For this review, take the finished solid that the model builds, in its own axes (mm). A direction names the side the tool comes from. Coordinates: 2 decimals unless noted, no trailing zeros. Order: outer loops, then holes, each group sorted by start corner. A loop starts at its lowest first (then second) coordinate and runs counter-clockwise, first axis right, second up. Notation, with made-up numbers: (58.25, -24) -> (107.25, -24) arc R19 cw to (107.25, -19) -> close; hole circle Ø4 at (25, 36.5). An arc over 180 degrees is marked (long way). Answer as a JSON object with one key per item and string values. Group by question number.
1) Wall thickness on L1, parallel to X at y = 16, z = 112; L2, parallel to Y at x = 186.75, z = 135.5; L3, parallel to Z at x = 184.25, y = 3: over which ranges is each line inside the solid? List them lowest first.
2) Add section A-A, the plane x = 185. Write out the cut boundary in (y, z).
3) Machinability: for faces 4 (the flat face through (182, 22, 130)), 5 (the flat face through (184, -17, 119)), 6 (the flat face through (185.6, -19.5, 129.3)), which of the approach directions +Z, -Z, +X, -X, +Y, -Y give a long, thin tool a straight path to every point of the face, cutting with its end or side? Answer none if there is none.
4) Draft analysis for pull direction Y (two halves, no side actions). For faces 1 (the flat face through (184, 17, 119)), 2 (the flat face through (182, -22, 130)), 3 (the flat face through (184, -21, 115.5)), state which applies: +Y half, -Y half, draft (parallel to the pull), parting line (faces both ways), or undercut.
5) Add section B-B, the plane z = 114. Write out the cut boundary in (x, y).
6) For pin 1 (1.2 mm diameter, centred on y = -16.5, z = 140, fed in from +X); pin 2 (0.8 mm diameter, centred on x = 186.5, z = 136.5, fed in from +Y); pin 3 (12 mm diameter, centred on y = 10, z = 142, fed in from +X); pin 4 (5.5 mm diameter, centred on x = 197, y = 16, fed in from -Z), all flat-tipped, find the tip position at first contact; note any pin that passes through.
7) Add section D-D, the plane z = 119.5. Write out the cut boundary in (x, y), then the cut area to 3 significant figures.
8) Add section C-C, the plane y = -16.5. Write out the cut boundary in (x, z).
from build123d import *

# Parameters (mm, degrees)
MOUNTING_FOOT_SKETCH_W      = 24
MOUNTING_FOOT_SKETCH_H      = 46
MOUNTING_FOOT_DEPTH         = 3
BACK_PLATE_SKETCH_W         = 3
BACK_PLATE_SKETCH_H         = 44
BACK_PLATE_DEPTH            = 31.5
CLIP_RAILS_DEPTH            = 30
TOP_RETAINING_RAIL_SKETCH_W = 6.1
TOP_RETAINING_RAIL_SKETCH_H = 40
TOP_RETAINING_RAIL_DEPTH    = 2
PCB_SUPPORT_SKETCH_R        = 2
PCB_SUPPORTS_DEPTH          = 3
MOUNTING_HOLES_SKETCH_R     = 1.7
MOUNTING_HOLES_DEPTH        = 3.2


with BuildPart() as part:
    # Mounting Foot Sketch → Mounting Foot (new body)
    with BuildSketch(Plane.XY.offset(111.5)):
        with Locations((190, 0)):
            Rectangle(MOUNTING_FOOT_SKETCH_W, MOUNTING_FOOT_SKETCH_H)
    extrude(amount=MOUNTING_FOOT_DEPTH)

    # Back Plate Sketch → Back Plate (add)
    with BuildSketch(Plane.XY.offset(114.5)):
        with Locations((179.5, 0)):
            Rectangle(BACK_PLATE_SKETCH_W, BACK_PLATE_SKETCH_H)
    extrude(amount=BACK_PLATE_DEPTH)

    # Clip Rail Sketch → Clip Rails (add)
    with BuildSketch(Plane.XY.offset(115.5)):
        Polygon((181, -22), (187.1, -22), (187.1, -19), (185.6, -19), (185.6, -20), (181, -20), align=None)
        Polygon((181, 20), (185.6, 20), (185.6, 19), (187.1, 19), (187.1, 22), (181, 22), align=None)
    extrude(amount=CLIP_RAILS_DEPTH)

    # Top Retaining Rail Sketch → Top Retaining Rail (add)
    with BuildSketch(Plane.XY.offset(143.5)):
        with Locations((184.05, 0)):
            Rectangle(TOP_RETAINING_RAIL_SKETCH_W, TOP_RETAINING_RAIL_SKETCH_H)
    extrude(amount=TOP_RETAINING_RAIL_DEPTH)

    # PCB Support Sketch → PCB Supports (add)
    with BuildSketch(Plane(origin=(181, 0, 0), x_dir=(0, 0, -1), z_dir=(1, 0, 0))):
        with Locations(Location((-119.5, -17, 0), (0, 0, 180))):
            Circle(PCB_SUPPORT_SKETCH_R)
        with Locations(Location((-140.5, -17, 0), (0, 0, 180))):
            Circle(PCB_SUPPORT_SKETCH_R)
        with Locations(Location((-119.5, 17, 0), (0, 0, 180))):
            Circle(PCB_SUPPORT_SKETCH_R)
        with Locations(Location((-140.5, 17, 0), (0, 0, 180))):
            Circle(PCB_SUPPORT_SKETCH_R)
    extrude(amount=PCB_SUPPORTS_DEPTH)

    # Mounting Holes Sketch → Mounting Holes (cut)
    with BuildSketch(Plane.XY.offset(111.4)):
        with Locations((185, -16)):
            Circle(MOUNTING_HOLES_SKETCH_R)
        with Locations((185, 16)):
            Circle(MOUNTING_HOLES_SKETCH_R)
        with Locations((197, -16)):
            Circle(MOUNTING_HOLES_SKETCH_R)
        with Locations((197, 16)):
            Circle(MOUNTING_HOLES_SKETCH_R)
    extrude(amount=MOUNTING_HOLES_DEPTH, mode=Mode.SUBTRACT)


solid = part.part
Output values:
{
 "1": {"L1": "x = 178 to 183.3, 186.7 to 195.3, 198.7 to 202", "L2": "y = -22 to -19, 19 to 22", "L3": "z = 111.5 to 114.5, 143.5 to 145.5"},
 "2": {"outline": "(-23, 111.5) -> (-17.7, 111.5) -> (-17.7, 114.5) -> (-23, 114.5) -> close; (-22, 115.5) -> (-20, 115.5) -> (-20, 143.5) -> (20, 143.5) -> (20, 115.5) -> (22, 115.5) -> (22, 145.5) -> (-22, 145.5) -> close; (-14.3, 111.5) -> (14.3, 111.5) -> (14.3, 114.5) -> (-14.3, 114.5) -> close; (17.7, 111.5) -> (23, 111.5) -> (23, 114.5) -> (17.7, 114.5) -> close"},
 "3": {"face 4": "+Z, +X, -X, +Y", "face 5": "+X", "face 6": "none"},
 "4": {"face 1": "undercut", "face 2": "-Y half", "face 3": "draft"},
 "5": {"outline": "(178, -23) -> (202, -23) -> (202, 23) -> (178, 23) -> close; hole circle Ø3.4 at (185, -16); hole circle Ø3.4 at (185, 16); hole circle Ø3.4 at (197, -16); hole circle Ø3.4 at (197, 16)"},
 "6": {"pin 1": "stops at x = 184", "pin 2": "stops at y = 22", "pin 3": "stops at x = 187.1", "pin 4": "stops at z = 111.5"},
 "7": {"outline": "(178, -22) -> (187.1, -22) -> (187.1, -19) -> (185.6, -19) -> (185.6, -20) -> (181, -20) -> (181, -19) -> (184, -19) -> (184, -15) -> (181, -15) -> (181, 15) -> (184, 15) -> (184, 19) -> (181, 19) -> (181, 20) -> (185.6, 20) -> (185.6, 19) -> (187.1, 19) -> (187.1, 22) -> (178, 22) -> close", "area": "183 mm²"},
 "8": {"outline": "(178, 111.5) -> (183.38, 111.5) -> (183.38, 114.5) -> (181, 114.5) -> (181, 117.56) -> (184, 117.56) -> (184, 121.44) -> (181, 121.44) -> (181, 138.56) -> (184, 138.56) -> (184, 142.44) -> (181, 142.44) -> (181, 143.5) -> (187.1, 143.5) -> (187.1, 145.5) -> (181, 145.5) -> (181, 146) -> (178, 146) -> close; (186.62, 111.5) -> (195.38, 111.5) -> (195.38, 114.5) -> (186.62, 114.5) -> close; (198.62, 111.5) -> (202, 111.5) -> (202, 114.5) -> (198.62, 114.5) -> close"}
}
